Build history of the part. All positions in model axes, mm. A direction names the side the tool comes from. Round coordinates to 2 decimals unless told otherwise and drop trailing zeros. Loops run counter-clockwise (first coordinate to the right, second up) from the corner with the lowest first, then second, coordinate; pieces in that order, holes last. Notation, with made-up numbers: M 37,69 L 78,69 A14 cw 78,90 Z; hole C 84,73.5 d6. An arc over 180 degrees is marked long. One line per item, written item: value.
Autodesk Inventor part; units mm, degrees
ref_plane "YZ Plane" through (0, 0, 0) normal (1, 0, 0) x (0, 1, 0)
ref_plane "XZ Plane" through (0, 0, 0) normal (0, 1, 0) x (-1, 0, 0)
ref_plane "XY Plane" through (0, 0, 0) normal (0, 0, 1) x (1, 0, 0)
sketch "Sketch1" plane through (0, 0, 0) normal (0, 0, 1) x (1, 0, 0)
  line L0 (0, 0) -> (240, 0)
  line L1 (240, 0) -> (240, 100)
  line L2 (240, 100) -> (0, 100)
  line L3 (0, 100) -> (0, 0)
  line L4 (70, 0) -> (170, 0)
  line L5 (170, 0) -> (170, -5.3)
  line L6 (170, -5.3) -> (70, -5.3)
  line L7 (70, -5.3) -> (70, 0)
  line L8 (70, 100) -> (170, 100)
  line L9 (170, 100) -> (170, 105.3)
  line L10 (170, 105.3) -> (70, 105.3)
  line L11 (70, 105.3) -> (70, 100)
  point P0 (0, 20)
  point P1 (170, 0)
  dimension "d0" = 240
  dimension "d1" = 100
  dimension "d2" = 100
  dimension "d3" = 5.3
  dimension "d8" = 70
  dimension "d9" = 5.3
extrude "Extrusion1" add sketch "Sketch1" along normal blind 5
properties part number "front"
Item 1: Wall check: line 1 along Y through (x, z) = (50, 4.55). Give the ranges that are in metal, low to high.
Check values:
line 1: y = 0 to 100
Item 2: Drop flat-ended pins along their axis: P1, Ø1.5, axis at y = 103, z = 2, coming from the -X side; P2, Ø1, axis at x = 28, y = 43.5, coming from the -Z side. Give the stop position or say it passes through.
Check values:
P1: stops at x = 70
P2: stops at z = 0
Item 3: Which spindle directions (+Z, -Z, +X, -X, +Y, -Y) get a long thin tool onto all of the face, cutting with end or side? Do faces 1 (the face through (205, 0, 2)), 2 (the face through (121, -5.3, 2)), 3 (the face through (205, 100, 2)), 4 (the face through (35, 0, 2)), 5 (the face through (70, 103, 2)). Say none if no direction does.
Check values:
face 1: +Z, -Z, +X, -Y
face 2: +Z, -Z, +X, -X, -Y
face 3: +Z, -Z, +X, +Y
face 4: +Z, -Z, -X, -Y
face 5: +Z, -Z, -X, +Y
Item 4: Slice it at A-A, the plane z = 3.7. Give the cut face in (x, y).
Check values:
outline: M 0,0 L 70,0 L 70,-5.3 L 170,-5.3 L 170,0 L 240,0 L 240,100 L 170,100 L 170,105.3 L 70,105.3 L 70,100 L 0,100 Z
Item 5: Slice it at B-B, the plane x = 23. Give the cut face in (y, z), and give its area (3 significant figures).
Check values:
outline: M 0,0 L 100,0 L 100,5 L 0,5 Z
area: 500 mm2
